```python
from build123d import *

# Parameters (mm, degrees)
BOSS_EXTRUDE1_DEPTH     = 1
SKETCH4_W               = 5.8
SKETCH4_H               = 5
BOSS_EXTRUDE2_DEPTH     = 1.5
CUT_EXTRUDE2_DEPTH      = 19.875882218
CUT_EXTRUDE2_DEPTH_BACK = 19.875882218
SKETCH3_R               = 2
FILLET2_SIZE            = 1
SKETCH11_R              = 2.5
CUT_EXTRUDE4_DEPTH      = 0.5


with BuildPart() as part:
    # Sketch1 → Boss-Extrude1 (new body)
    with BuildSketch(Plane.XY):
        with BuildLine():
            Line((-3, -6.860294118), (3, -6.860294118))
            ThreePointArc((3, -6.860294118), (4.414213562, -6.27450768), (5, -4.860294118))
            Line((5, -4.860294118), (5, 3.139705882))
            Line((5, 3.139705882), (3.115711504, 17.271869602))
            ThreePointArc((3.115711504, 17.271869602), (2.783208235, 17.89209), (2.124483603, 18.139705882))
            Line((2.124483603, 18.139705882), (-2.124483603, 18.139705882))
            ThreePointArc((-2.124483603, 18.139705882), (-2.783208235, 17.89209), (-3.115711504, 17.271869602))
            Line((-3.115711504, 17.271869602), (-5, 3.139705882))
            Line((-5, 3.139705882), (-5, -4.860294118))
            ThreePointArc((-5, -4.860294118), (-4.414213562, -6.27450768), (-3, -6.860294118))
        make_face()
    extrude(amount=BOSS_EXTRUDE1_DEPTH)

    # Sketch4 → Boss-Extrude2 (add)
    with BuildSketch(Plane.XY.offset(1)):
        with Locations((0, -4.360294118)):
            Rectangle(SKETCH4_W, SKETCH4_H)
    extrude(amount=BOSS_EXTRUDE2_DEPTH)

    # Sketch3 → Cut-Extrude2 (cut, two sides: drawn at the far end of the back side and taken through both)
    with BuildSketch(Plane.XY.offset(1).offset(-CUT_EXTRUDE2_DEPTH_BACK)):
        with Locations((0, -1.860294118)):
            Circle(SKETCH3_R)
    extrude(amount=CUT_EXTRUDE2_DEPTH + CUT_EXTRUDE2_DEPTH_BACK, mode=Mode.SUBTRACT)

    # Sketch10 → Revolve1 (revolve)
    with BuildSketch(Plane.ZY):
        with BuildLine():
            Line((3, 13.139705882), (1, 13.139705882))
            Line((1, 13.139705882), (1, 15.164832594))
            add(Edge.make_bspline(
                [(1, 15.164832594), (1.003638123, 14.768281169), (2.909332007, 13.597450134), (3, 13.139705882)],
                knots=[0, 0, 0, 0, 1, 1, 1, 1], degree=3))
        make_face()
    revolve(axis=Axis((0, 13.139705882, 3), (0, 0, -1)))

    # Fillet2
    # a fillet whose section is not a circle: 1 mm, written as the material it takes off along each edge
    with BuildSketch(Plane(origin=(2.9, -9.360294118, 2.5), x_dir=(0, 0, -1), z_dir=(0, 1, 0)), Plane(origin=(-2.9, 0.639705882, 2.5), x_dir=(0, 0, -1), z_dir=(0, -1, 0))) as fillet2_piece_1:
        with BuildLine():
            add(Edge.make_bspline([(FILLET2_SIZE, 0), (FILLET2_SIZE * 0.831801948466, 0), (FILLET2_SIZE * 0.663603896932, 0), (FILLET2_SIZE * 0.292893218813, FILLET2_SIZE * 0.0716919198361), (FILLET2_SIZE * 0.0716919198361, FILLET2_SIZE * 0.292893218813), (0, FILLET2_SIZE * 0.663603896932), (0, FILLET2_SIZE * 0.831801948466), (0, FILLET2_SIZE)], knots=[0, 0, 0, 0, 0, 0, 0.5, 0.5, 1, 1, 1, 1, 1, 1], degree=5))
            Line((0, FILLET2_SIZE), (0, 0))
            Line((0, 0), (FILLET2_SIZE, 0))
        make_face()
    fillet2_piece_1_solid = extrude(amount=10, mode=Mode.PRIVATE)
    with BuildSketch(Plane(origin=(2.9, -6.860294118, 1), x_dir=(-1, 0, 0), z_dir=(0, 0, 1))) as fillet2_piece_2:
        with BuildLine():
            add(Edge.make_bspline([(FILLET2_SIZE, 0), (FILLET2_SIZE * 0.831801948466, 0), (FILLET2_SIZE * 0.663603896932, 0), (FILLET2_SIZE * 0.292893218813, -FILLET2_SIZE * 0.0716919198361), (FILLET2_SIZE * 0.0716919198361, -FILLET2_SIZE * 0.292893218813), (0, -FILLET2_SIZE * 0.663603896932), (0, -FILLET2_SIZE * 0.831801948466), (0, -FILLET2_SIZE)], knots=[0, 0, 0, 0, 0, 0, 0.5, 0.5, 1, 1, 1, 1, 1, 1], degree=5))
            Line((0, -FILLET2_SIZE), (0, 0))
            Line((0, 0), (FILLET2_SIZE, 0))
        make_face()
    fillet2_piece_2_solid = extrude(amount=4, mode=Mode.PRIVATE)
    with BuildSketch(Plane(origin=(-2.9, -6.860294118, 1), x_dir=(1, 0, 0), z_dir=(0, 0, 1))) as fillet2_piece_3:
        with BuildLine():
            add(Edge.make_bspline([(FILLET2_SIZE, 0), (FILLET2_SIZE * 0.831801948466, 0), (FILLET2_SIZE * 0.663603896932, 0), (FILLET2_SIZE * 0.292893218813, FILLET2_SIZE * 0.0716919198361), (FILLET2_SIZE * 0.0716919198361, FILLET2_SIZE * 0.292893218813), (0, FILLET2_SIZE * 0.663603896932), (0, FILLET2_SIZE * 0.831801948466), (0, FILLET2_SIZE)], knots=[0, 0, 0, 0, 0, 0, 0.5, 0.5, 1, 1, 1, 1, 1, 1], degree=5))
            Line((0, FILLET2_SIZE), (0, 0))
            Line((0, 0), (FILLET2_SIZE, 0))
        make_face()
    fillet2_piece_3_solid = extrude(amount=4, mode=Mode.PRIVATE)
    add([fillet2_piece_1_solid, fillet2_piece_2_solid, fillet2_piece_3_solid], mode=Mode.SUBTRACT)

    # Sketch11 → Cut-Extrude4 (cut)
    with BuildSketch(Plane.XY.offset(1)):
        with Locations((0, 18.139705882)):
            Circle(SKETCH11_R)
    extrude(amount=-CUT_EXTRUDE4_DEPTH, mode=Mode.SUBTRACT)


solid = part.part
```
Could you check a few things on this model? Use its own coordinates, in mm. A direction names the side the tool comes from. Round coordinates to 2 decimals unless told otherwise and drop trailing zeros. Order: outer loops, then holes, each group sorted by start corner. A loop starts at its lowest first (then second) coordinate and runs counter-clockwise, first axis right, second up. Notation, with made-up numbers: (79, -13.5) -> (112, -13.5) arc R30 cw to (112, 21.5) -> close; hole circle Ø3 at (-23.5, 69). An arc over 180 degrees is marked (long way). One line per question, with ' | ' between items.
Q1. If we section it at A-A on z = 0.75: Write out the boundary of the cut face in (x, y).
Computed values:
outline: (-5, -4.86) arc R2 ccw to (-3, -6.86) -> (3, -6.86) arc R2 ccw to (5, -4.86) -> (5, 3.14) -> (3.12, 17.27) arc R1 ccw to (2.5, 18.07) arc R2.5 cw to (-2.5, 18.07) arc R1 ccw to (-3.12, 17.27) -> (-5, 3.14) -> close; hole circle Ø4 at (0, -1.86)
Q2. If I drill on line 1 (Y direction, x = 0, z = 0.6); line 2 (Z direction, x = 3.25, y = 15.25); line 3 (X direction, y = -0.5, z = 0.8), over which ranges is the centre line in solid material (lowest first)? Write a range as from..to.
Computed values:
line 1: -6.86..-3.86, 0.14..15.64 | line 2: 0..1 | line 3: -5..-1.47, 1.47..5
Q3. I'm going to push flat-ended pins straight in: pin 1 (1.1 mm diameter, centred on x = -0.5, y = -4.5, fed in from +Z); pin 2 (0.5 mm diameter, centred on x = 2.5, z = 1.5, fed in from +Y); pin 3 (0.8 mm diameter, centred on x = 1, y = 17.5, fed in from +Z). Where does each tip first touch, or does it pass through?
Computed values:
pin 1: z = 2.5 | pin 2: y = -1.86 | pin 3: z = 0.5
Q4. Which directions (+Z, -Z, +X, -X, +Y, -Y) give clear straight access to the entire face, cutting with the end or side of a thin tool? Please do faces 4 (the face through (0, 6, 1)), 5 (the face through (-2.5, -1.86, 1.7)), 6 (the face through (-0.434, -3.813, 0.955)), 7 (the face through (2.791, 17.885, 0.493)), 8 (the face through (-0.05, 15.64, 0.75)).
Computed values:
face 4: +Z | face 5: +Z, +X, -X, +Y | face 6: +Z, -Z | face 7: +Z, -Z, +X, +Y | face 8: +Z, +Y
Q5. If we section it at C-C on x = 3.5: Write out the boundary of the cut face in (y, z), plus the area to 3 significant figures.
Computed values:
outline: (-6.8, 0) -> (14.39, 0) -> (14.39, 1) -> (-6.8, 1) -> close | area: 21.2 mm²
Q6. We'd pull the mould along X, two halves only. Please class faces 1 (the face through (0, -5, 2.5)), 2 (the face through (0, 17, 0.5)), 3 (the face through (-4.43, -6.26, 0.49)): released by +X, released by -X, zero draft, split by the parting line, or undercut.
Computed values:
face 1: zero draft | face 2: undercut | face 3: released by -X
Q7. If we section it at B-B on y = 2.5: Write out the boundary of the cut face in (x, z).
Computed values:
outline: (-5, 0) -> (5, 0) -> (5, 1) -> (-5, 1) -> close
